Geometry: final body of the model. Coordinates: model frame, mm. A direction names the side the tool comes from. Give positions to 0.01 mm unless a question says otherwise; leave off trailing zeros. Loops run counter-clockwise (first coordinate to the right, second up) from the corner with the lowest first, then second, coordinate; pieces in that order, holes last.
Autodesk Inventor part; units mm, degrees
ref_plane "YZ Plane" through (0, 0, 0) normal (1, 0, 0) x (0, 1, 0)
ref_plane "XZ Plane" through (0, 0, 0) normal (0, 1, 0) x (-1, 0, 0)
ref_plane "XY Plane" through (0, 0, 0) normal (0, 0, 1) x (1, 0, 0)
sketch "Sketch1" plane through (0, 0, 0) normal (0, 0, 1) x (1, 0, 0)
  line L0 (0, 0) -> (0, 7.239) construction
  line L1 (0, 0) -> (6.2692, 3.6195) construction
  line L2 (0, 0) -> (6.2692, -3.6195) construction
  line L3 (0, 0) -> (0, -7.239) construction
  line L4 (0, 0) -> (-6.2692, -3.6195) construction
  line L5 (0, 0) -> (-6.2692, 3.6195) construction
  line L6 (0, 7.239) -> (6.2692, 3.6195)
  line L7 (6.2692, 3.6195) -> (6.2692, -3.6195)
  line L8 (6.2692, -3.6195) -> (0, -7.239)
  line L9 (0, -7.239) -> (-6.2692, -3.6195)
  line L10 (-6.2692, -3.6195) -> (-6.2692, 3.6195)
  line L11 (-6.2692, 3.6195) -> (0, 7.239)
  circle A0 centre (0, 7.239) radius 2.3813
  circle A1 centre (6.2692, -3.6195) radius 2.3813
  circle A2 centre (-6.2692, -3.6195) radius 2.3813
  circle A3 centre (0, 0) radius 31.75
  line L12 (-2.3813, 7.239) -> (-2.3813, 5.8642)
  line L13 (2.3813, 7.239) -> (2.3812, 5.8642)
  line L14 (-2.3813, 7.239) -> (2.3813, 7.239)
  line L15 (-2.3813, 5.8642) -> (2.3812, 5.8642)
  line L16 (7.4598, -1.5573) -> (6.2692, -0.8699)
  line L17 (5.0785, -5.6817) -> (3.8879, -4.9943)
  line L18 (6.2692, -0.8699) -> (3.8879, -4.9943)
  line L19 (7.4598, -1.5573) -> (5.0785, -5.6817)
  line L20 (-7.4598, -1.5573) -> (-6.2692, -0.8699)
  line L21 (-5.0785, -5.6817) -> (-3.8879, -4.9943)
  line L22 (-7.4598, -1.5573) -> (-5.0785, -5.6817)
  line L23 (-3.8879, -4.9943) -> (-6.2692, -0.8699)
  dimension "d0" = 7.239
  dimension "d1" = 60
  dimension "d2" = 60
  dimension "d3" = 4.7625
  dimension "d4" = 4.7625
  dimension "d5" = 4.7625
  dimension "d6" = 63.5
extrude "Extrusion1" add sketch "Sketch1" along normal blind 12.7 contours L6 A0 L13 | L16 A1 L7 | A0 L11 L12 | A1 L17 L8 | L10 A2 L20 | L21 A2 L9 | A3
extrude "Extrusion2" cut sketch "Sketch1" along normal blind 12.7 contours L6 A0 L13 | L6 L7 L18 A1 L8 L9 L23 A2 L10 L11 L15 A0 | L6 L14 A0 | A0 L15 | L7 A1 L18 | L11 A0 L14 | A0 L11 L12 | L7 L8 A1 L18 | L18 A1 | A1 L8 L18 | L23 A2 L10 | A2 L23 L9 L10 | A2 L23 | L9 A2 L23
extrude "Extrusion3" cut sketch "Sketch1" along normal blind 12.7 contours L16 A1 L7 | A1 L19 L7 | A1 L19 | L19 A1 L8 | A1 L17 L8
extrude "Extrusion4" cut sketch "Sketch1" along normal through all contours L10 A2 L20 | L10 L22 A2 | L21 A2 L9 | L9 A2 L22
equation "\"d4\" = d3"
equation "\"d5\" = d3"
properties part number "augmented gear v3"
Item 1: Section query C-C on x = 26.5. Return loops of the section in (y, z).
Values follow:
outline: (-17.49, 0) - (17.49, 0) - (17.49, 12.7) - (-17.49, 12.7) - close
Item 2: Section query A-A on y = 0. Return loops of the section in (x, z).
Values follow:
outline: (-31.75, 0) - (-6.27, 0) - (-6.27, 12.7) - (-31.75, 12.7) - close; (6.27, 0) - (31.75, 0) - (31.75, 12.7) - (6.27, 12.7) - close
Item 3: Draft query along X for faces 3 (the face through (7, 0, 0)), 4 (the face through (-1.92, -6.13, 6.26)), 5 (the face through (-6.883, 30.995, 6.261)). Return one class per face: +X half, -X half, draft (parallel to the pull), parting line (faces both ways), or undercut.
Values follow:
face 3: draft
face 4: undercut
face 5: parting line
Item 4: Ray query, probe 1 along X at (y, z) = (1, 5.5); probe 2 along Y at (x, z) = (7.5, 6.75); probe 3 along X at (y, z) = (-2.5, 10). Return the intervals inside material, ascending.
Values follow:
probe 1: x = -31.73 to -6.27, 6.27 to 31.73
probe 2: y = -30.85 to -5.66, -1.58 to 30.85
probe 3: x = -31.65 to -8.37, 8.37 to 31.65
Item 5: Pin query (flat end, axial travel): pin 1 (1.1 mm diameter, centred on y = 6.5, z = 6.5, fed in from +X); pin 2 (5 mm diameter, centred on y = 19, z = 2, fed in from +X); pin 3 (1.5 mm diameter, centred on y = 6.5, z = 7.5, fed in from -X) (3 decimals). Return the tip coordinate at first contact, or that it passes through.
Values follow:
pin 1: stops at x = 31.19
pin 2: stops at x = 27.13
pin 3: stops at x = -31.225
Item 6: Section query B-B on z = 11.25. Return loops of the section in (x, y).
Values follow:
outline: circle Ø63.5 at (0, 0); hole (-7.46, -1.56) arc R2.38 ccw to (-5.08, -5.68) - (-3.89, -4.99) - (0, -7.24) - (3.89, -4.99) - (5.08, -5.68) arc R2.38 ccw to (7.46, -1.56) - (6.27, -0.87) - (6.27, 3.62) - (2.38, 5.86) - (2.38, 7.24) arc R2.38 ccw to (-2.38, 7.24) - (-2.38, 5.86) - (-6.27, 3.62) - (-6.27, -0.87) - close
Item 7: Set-up query: faces 1 (the face through (7, 0, 12.7)), 2 (the face through (6.269, 1, 6)). Return all of +Z, -Z, +X, -X, +Y, -Y with unobstructed straight access to the full face (end or side cutting, diameter ignored); none if empty.
Values follow:
face 1: +Z, +X, -X, +Y, -Y
face 2: +Z, -Z
Item 8: Section query D-D on y = -22.5. Return loops of the section in (x, z).
Values follow:
outline: (-22.4, 0) - (22.4, 0) - (22.4, 12.7) - (-22.4, 12.7) - close
